Work out the finished part from the listing and answer in its coordinate system (mm). A direction names the side the tool comes from. Coordinates: 2 decimals unless noted, no trailing zeros. Order: outer loops, then holes, each group sorted by start corner. A loop starts at its lowest first (then second) coordinate and runs counter-clockwise, first axis right, second up. Notation, with made-up numbers: M -9.75,36.25 L 25.25,36.25 A22 ccw 25.25,64.25 Z; hole C 71.25,-18.75 d9. An arc over 180 degrees is marked long. Write item = value, one per line. Start each with the question number.
Q1. Find section C-C on z = -7.5. Give the vertices of the cut face in (x, y).
Q2. Find section B-B on y = 92.5. Give the vertices of the cut face in (x, z), and give its area (3 significant figures).
Q3. Straight lines are drawn through the part: line 1 along X through (y, z) = (5.5, 1); line 2 along Y through (x, z) = (-1, 26); line 3 along Y through (x, z) = (-8, -74.5). For each, find the intervals that lie inside material, in ascending order.
Q4. Find section D-D on y = 29.5. Give the vertices of the cut face in (x, z), and give its area (3 significant figures).
Q5. A tool of negligible diameter and unlimited length cuts with its end or side. For faces 1 (the cylindrical face through (-32.297, 89.86, -83.986)), 2 (the flat face through (0, 75, 0)), from which of +Z, -Z, +X, -X, +Y, -Y can it reach the whole face along a straight path? Write none if from no direction.
Q6. Find section A-A on x = 0. Give the vertices of the cut face in (y, z), and give its area (3 significant figures).
Q7. Each of these flat-tipped pins is pushed along its axis until it touches: P1, Ø12, axis at x = -11, y = 69, coming from the +Z side; P2, Ø1.5, axis at x = -20, y = 30.5, coming from the -Z side; P3, Ø3, axis at y = 51.5, z = -24.5, coming from the -X side. Where does it stop, or does it pass through?
```python
from build123d import *

# Parameters (mm, degrees)
SKETCH1_R           = 38
BOSS_EXTRUDE1_DEPTH = 80
SKETCH2_R           = 29
CUT_EXTRUDE1_DEPTH  = 75
BOSS_EXTRUDE2_DEPTH = 20


with BuildPart() as part:
    # Sketch1 → Boss-Extrude1 (new body)
    with BuildSketch(Plane(origin=(0, 0, 0), x_dir=(1, 0, 0), z_dir=(0, 1, 0))):
        with Locations(Location((0, 0, 0), (0, 0, 270))):
            Circle(SKETCH1_R)
    extrude(amount=BOSS_EXTRUDE1_DEPTH)

    # Sketch2 → Cut-Extrude1 (cut)
    with BuildSketch(Plane.XZ):
        with Locations(Location((0, 0, 0), (0, 0, 270))):
            Circle(SKETCH2_R)
    extrude(amount=-CUT_EXTRUDE1_DEPTH, mode=Mode.SUBTRACT)

    # Sketch3 → Boss-Extrude2 (add)
    with BuildSketch(Plane(origin=(0, 80, 0), x_dir=(1, 0, 0), z_dir=(0, 1, 0))):
        with BuildLine():
            Line((18, -90), (-18, -90))
            ThreePointArc((-18, -90), (-32.142135624, -84.142135624), (-38, -70))
            Line((-38, -70), (-38, 70))
            ThreePointArc((-38, 70), (-32.142135624, 84.142135624), (-18, 90))
            Line((-18, 90), (18, 90))
            ThreePointArc((18, 90), (32.142135624, 84.142135624), (38, 70))
            Line((38, 70), (38, -70))
            ThreePointArc((38, -70), (32.142135624, -84.142135624), (18, -90))
        make_face()
    extrude(amount=BOSS_EXTRUDE2_DEPTH)


solid = part.part
```
Findings below:
q1.outline = M -38,80 L -37.25,80 L -37.25,0 L -28.01,0 L -28.01,75 L 28.01,75 L 28.01,0 L 37.25,0 L 37.25,80 L 38,80 L 38,100 L -38,100 Z
q2.outline = M -38,-70 A20 ccw -18,-90 L 18,-90 A20 ccw 38,-70 L 38,70 A20 ccw 18,90 L -18,90 A20 ccw -38,70 Z
q2.area = 13,300 mm^2
q3.line_1 = -37.99 to -28.98, 28.98 to 37.99
q3.line_2 = 75 to 100
q3.line_3 = 80 to 100
q4.outline = C 0,0 d76; hole C 0,0 d58
q4.area = 1,890 mm^2
q5.face_1 = -Z, -X, +Y, -Y
q5.face_2 = -Y
q6.outline = M 0,-38 L 80,-38 L 80,-90 L 100,-90 L 100,90 L 80,90 L 80,38 L 0,38 L 0,29 L 75,29 L 75,-29 L 0,-29 Z
q6.area = 5,330 mm^2
q7.P1 = 37.67
q7.P2 = -32.76
q7.P3 = -30.25
